Geometry check sheet. Reference: the model listing, model coordinates, mm. A direction names the side the tool comes from. Round coordinates to 2 decimals unless told otherwise and drop trailing zeros. Order: outer loops, then holes, each group sorted by start corner. A loop starts at its lowest first (then second) coordinate and runs counter-clockwise, first axis right, second up.
(1) Sectioned sample at B-B (x = 22). Record the boundary of the cut face in (y, z), plus the area to 3 significant figures.
(2) Go/stop test with flat-tipped pins: pin 1 (3 mm diameter, centred on x = 33, z = 0, fed in from -Y); pin 2 (4 mm diameter, centred on x = 6, z = 0, fed in from +Y). Record where each tip stops, or that it passes through.
(3) Sectioned sample at D-D (z = 2.75). Record the boundary of the cut face in (x, y).
(4) Material ranges on line 1 along X through (y, z) = (18.85, 0); line 2 along Z through (x, y) = (33, 20); line 3 along Y through (x, z) = (10.5, 0.75), recorded low to high.
(5) Set-up check for faces 5 (the face through (0, 0, 0)), 6 (the face through (34.8, -16.22, -0.07)): record each of +Z, -Z, +X, -X, +Y, -Y from which the full face is reachable in a straight line by a thin tool's end or side.
(6) Sectioned sample at C-C (y = -3.5). Record the boundary of the cut face in (x, z), plus the area to 3 significant figures.
(7) Release check for a two-part mould opening along Z. For faces 1 (the face through (37, 0, -5)), 2 (the face through (4.476, -19.374, -0.632)), 3 (the face through (19, -17.35, 0)), 4 (the face through (4.35, 19.37, 0.07)) record: +Z half, -Z half, draft (parallel to the pull), parting line (faces both ways), or undercut.
(8) Sectioned sample at A-A (z = 0). Record the boundary of the cut face in (x, y).
from build123d import *

# Parameters (mm, degrees)
ESQUISSE1_W               = 39
ESQUISSE1_H               = 10
EXTRUSION1_DEPTH          = 22.35
TROU_TARAUD_M4X0_71_D     = 3.3
TROU_TARAUD_M4X0_71_DEPTH = 10.1
TROU_TARAUD_M4X0_71_TIP   = 0.991420021
TROU_TARAUD_M4X0_72_D     = 3.3
TROU_TARAUD_M4X0_72_DEPTH = 10.1
TROU_TARAUD_M4X0_72_TIP   = 0.991420021
ENL_V_MAT_EXTRU_1_DEPTH   = 47.049131371


with BuildPart() as part:
    # Esquisse1 → Extrusion1 (new, symmetric)
    with BuildSketch(Plane(origin=(0, 0, 0), x_dir=(1, 0, 0), z_dir=(0, 1, 0))):
        with Locations((19.5, 0)):
            Rectangle(ESQUISSE1_W, ESQUISSE1_H)
    extrude(amount=EXTRUSION1_DEPTH, both=True)

    # Trou taraudé M4x0.71
    with Locations(Plane.XZ.offset(22.35)):
        with Locations((33, 0), (6, 0)):
            Hole(TROU_TARAUD_M4X0_71_D / 2, depth=TROU_TARAUD_M4X0_71_DEPTH)
            with Locations((0, 0, -(TROU_TARAUD_M4X0_71_DEPTH + TROU_TARAUD_M4X0_71_TIP / 2))):  # 118° drill point
                Cone(0, TROU_TARAUD_M4X0_71_D / 2, TROU_TARAUD_M4X0_71_TIP, mode=Mode.SUBTRACT)

    # Trou taraudé M4x0.72
    with Locations(Plane(origin=(0, 22.35, 0), x_dir=(-1, 0, 0), z_dir=(0, 1, 0))):
        with Locations((-6, 0), (-33, 0)):
            Hole(TROU_TARAUD_M4X0_72_D / 2, depth=TROU_TARAUD_M4X0_72_DEPTH)
            with Locations((0, 0, -(TROU_TARAUD_M4X0_72_DEPTH + TROU_TARAUD_M4X0_72_TIP / 2))):  # 118° drill point
                Cone(0, TROU_TARAUD_M4X0_72_D / 2, TROU_TARAUD_M4X0_72_TIP, mode=Mode.SUBTRACT)

    # Esquisse8 → Enlèv. mat.-Extru.1 (cut, through all)
    with BuildSketch(Plane(origin=(0, 0, -5), x_dir=(-1, 0, 0), z_dir=(0, 0, -1))):
        with BuildLine():
            Line((-33, 17.35), (-6, 17.35))
            ThreePointArc((-6, 17.35), (-4.585786438, 16.764213562), (-4, 15.35))
            Line((-4, 15.35), (-4, -15.35))
            ThreePointArc((-4, -15.35), (-4.585786438, -16.764213562), (-6, -17.35))
            Line((-6, -17.35), (-33, -17.35))
            ThreePointArc((-33, -17.35), (-34.414213562, -16.764213562), (-35, -15.35))
            Line((-35, -15.35), (-35, 15.35))
            ThreePointArc((-35, 15.35), (-34.414213562, 16.764213562), (-33, 17.35))
        make_face()
    extrude(amount=-ENL_V_MAT_EXTRU_1_DEPTH, mode=Mode.SUBTRACT)


solid = part.part
Answer below:
1. outline: (-22.35, -5) - (-17.35, -5) - (-17.35, 5) - (-22.35, 5) - close; (17.35, -5) - (22.35, -5) - (22.35, 5) - (17.35, 5) - close
1. area: 100 mm2
2. pin 1: passes through
2. pin 2: stops at y = 22.35
3. outline: (0, -22.35) - (39, -22.35) - (39, 22.35) - (0, 22.35) - close; hole (4, -15.35) arc R2 ccw to (6, -17.35) - (33, -17.35) arc R2 ccw to (35, -15.35) - (35, 15.35) arc R2 ccw to (33, 17.35) - (6, 17.35) arc R2 ccw to (4, 15.35) - close
4. line 1: x = 0 to 4.35, 7.65 to 31.35, 34.65 to 39
4. line 2: z = -5 to -1.65, 1.65 to 5
4. line 3: y = -22.35 to -17.35, 17.35 to 22.35
5. face 5: +Z, -Z, -X, +Y, -Y
5. face 6: +Z, -Z
6. outline: (0, -5) - (4, -5) - (4, 5) - (0, 5) - close; (35, -5) - (39, -5) - (39, 5) - (35, 5) - close
6. area: 80.0 mm2
7. face 1: -Z half
7. face 2: undercut
7. face 3: draft
7. face 4: undercut
8. outline: (0, -22.35) - (4.35, -22.35) - (4.35, -16.48) arc R2 cw to (4, -15.35) - (4, 15.35) arc R2 cw to (4.35, 16.48) - (4.35, 22.35) - (0, 22.35) - close; (7.65, -22.35) - (31.35, -22.35) - (31.35, -17.35) - (7.65, -17.35) - close; (7.65, 17.35) - (31.35, 17.35) - (31.35, 22.35) - (7.65, 22.35) - close; (34.65, -22.35) - (39, -22.35) - (39, 22.35) - (34.65, 22.35) - (34.65, 16.48) arc R2 cw to (35, 15.35) - (35, -15.35) arc R2 cw to (34.65, -16.48) - close
